from build123d import *

# Parameters (mm, degrees)
F2_R = 3.6259131904
F4_R = 5.08
F5_R = 5.08


# Not quite as in the source:
# - a fillet or chamfer that OpenCascade refuses, or shapes differently, is made with other operations: its cross-section is extruded or revolved along the edge and cut away or added


with BuildPart() as f1:
    # F0 (on Front) → F1 (revolve)
    with BuildSketch(Plane.XZ):
        with BuildLine():
            Line((0, -74.6885836124), (35.6496162713, -74.6885836124))
            Line((35.6496162713, -74.6885836124), (35.6496162713, -67.5909221172))
            Line((35.6496162713, -67.5909221172), (31.4555428922, -64.3647164106))
            Line((31.4555428922, -64.3647164106), (35.3054043443, -59.3598894102))
            Line((35.3054043443, -59.3598894102), (18.550703302, -54.0408417583))
            Line((18.550703302, -54.0408417583), (18.550703302, -45.9753163159))
            Line((18.550703302, -45.9753163159), (9.1946963221, -43.0717244744))
            Line((9.1946963221, -43.0717244744), (9.1946963221, 0))
            Line((9.1946963221, 0), (37.2865381299, 3.8790097637))
            Line((37.2865381299, 3.8790097637), (12.0982844383, 11.773836799))
            Line((12.0982844383, 11.773836799), (12.0982844383, 12.354565))
            ThreePointArc((12.0982844383, 12.354565), (18.8461202348, 34.6279388467), (0, 48.2829826967))
            Line((0, 48.2829826967), (0, -74.6885836124))
        make_face()
    revolve(axis=Axis((0, 0, -13.2028004579), (0, 0, 1)))

    # F2
    f2_edges = [f1.edges().sort_by_distance(p)[0] for p in [
        (-37.286538, 0, 3.87901),
    ]]
    fillet(f2_edges, radius=F2_R)

    # F3: fillet of radius 5.08 on 1 edges, made by hand

    # F3_s1 → F3_t2 (revolve, cut)
    with BuildSketch(Plane.XZ):
        with BuildLine():
            ThreePointArc((28.4786431175, -57.1926249402), (31.6334069722, -60.0870384375), (31.4555428922, -64.3647164106))
            Line((31.4555428922, -64.3647164106), (35.3054043443, -59.3598894102))
            Line((35.3054043443, -59.3598894102), (28.4786431175, -57.1926249402))
        make_face()
    revolve(axis=Axis((0, 0, -59.3598894102), (0, 0, 1)), mode=Mode.SUBTRACT)

    # F4
    f4_edges = [f1.edges().sort_by_distance(p)[0] for p in [
        (-35.649616, 0, -67.590922),
    ]]
    fillet(f4_edges, radius=F4_R)

    # F5
    f5_edges = [f1.edges().sort_by_distance(p)[0] for p in [
        (-18.550703, 0, -45.975316),
    ]]
    fillet(f5_edges, radius=F5_R)


solid = f1.part
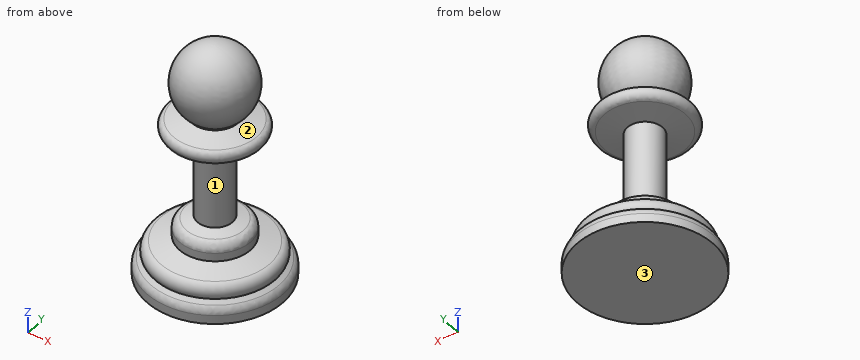
Geometry: final body of the model. Coordinates: model frame, mm. Face numbers are marked on the shaded views. Give positions to 0.01 mm unless a question says otherwise; leave off trailing zeros. Answer in a Markdown table with one row per item. Add a question column.
(1) Mould query, pull axis Z, two halves, no side actions, for the marked faces 1, 2 and 3. Classes: +Z half, -Z half, draft (parallel to the pull), parting line (faces both ways), or undercut.
(2) First-contact query: pin 1 (6 mm diameter, centred on x = 19.5, z = 7, fed in from +Y); pin 2 (4 mm diameter, centred on x = -11.5, y = -4, fed in from +Z); pin 3 (2 mm diameter, centred on x = -22, y = 5.5, fed in from +Z). Flat tips, straight axial feed; report the tip coordinate or a pass-through.
(3) Ray query, line 1 (Z direction, x = 8, y = -5); line 2 (Y direction, x = -3, z = -50.5); line 3 (X direction, y = 3, z = 35). Return the intervals inside material, ascending.
Result set:
| question | item | result |
|---|---|---|
| 1 | face 1 | undercut |
| 1 | face 2 | undercut |
| 1 | face 3 | -Z half |
| 2 | pin 1 | stops at y = 17.7 |
| 2 | pin 2 | stops at z = 45.41 |
| 2 | pin 3 | stops at z = 8.77 |
| 3 | line 1 | z = -74.69 to -43.15, 0.03 to 45.84 |
| 3 | line 2 | y = -18.31 to 18.31 |
| 3 | line 3 | x = -18.47 to 18.47 |
